Build history of the part. All positions in model axes, mm. Give positions to 0.01 mm unless a question says otherwise; leave off trailing zeros. Order: outer loops, then holes, each group sorted by start corner. A loop starts at its lowest first (then second) coordinate and runs counter-clockwise, first axis right, second up. Notation, with made-up numbers: (48, 31.25) - (91, 31.25) arc R5 cw to (91, 40.25) - close; hole circle Ø9 at (-36.75, 83.5). An arc over 180 degrees is marked (long way). Use a Markdown table: item, result. Add a question column.
(1) Slice it at D-D (x = 6). Write the cut outline in (y, z), then the cut area to 3 significant figures.
(2) Wall check: line 1 (Y direction, x = 0, z = -102.05); line 2 (X direction, y = 4.5, z = -101.05); line 3 (Y direction, x = -0.5, z = -100.25). Give the ranges that are in metal, low to high.
(3) Slice it at A-A (y = 0). Write the cut outline in (x, z), then the cut area to 3 significant figures.
(4) Mould opens along X. For faces 1 (the face through (11.444, -22.002, -102.028)), 2 (the face through (11, 6, -100)), 3 (the face through (14.5, 0, -102)) say: +X half, -X half, draft (parallel to the pull), parting line (faces both ways), or undercut.
(5) Slice it at C-C (y = -10). Write the cut outline in (x, z).
(6) Flat gauge pins, fed straight in: pin 1 (4 mm diameter, centred on x = 0, y = -16, fed in from +Z); pin 2 (2.5 mm diameter, centred on x = -16, y = 0, fed in from -Z); pin 3 (1.5 mm diameter, centred on x = -8, z = -102, fed in from -Y); pin 4 (2 mm diameter, centred on x = 10, z = -100.5, fed in from +Y). Where does each tip first touch, or does it go through?
from build123d import *

# Parameters (mm, degrees)
CYLINDER275_R               = 1.5
CYLINDER275_DEPTH           = 16
CYLINDER275_PLACEMENT_ANGLE = 67.5
CYLINDER273_R               = 1.5
CYLINDER273_DEPTH           = 16
CYLINDER273_PLACEMENT_ANGLE = 22.5
CYLINDER274_R               = 1.5
CYLINDER274_DEPTH           = 16
CYLINDER274_PLACEMENT_ANGLE = 112.5
CYLINDER272_R               = 1.5
CYLINDER272_DEPTH           = 16
CYLINDER272_PLACEMENT_ANGLE = 202.5
TUBE030_R                   = 24.8
TUBE030_R_2                 = 12
TUBE030_DEPTH               = 4


with BuildPart() as obj1:
    # Cylinder275 → Cylinder275 (new body)
    with BuildSketch(Plane.XY):
        Circle(CYLINDER275_R)
    extrude(amount=CYLINDER275_DEPTH)


with BuildPart() as obj1_1:
    # Cylinder275 placement: moved
    add(obj1.part.moved(Location((0, 16, 2))).rotate(Axis((0, 16, 2), (0, 0, -1)), CYLINDER275_PLACEMENT_ANGLE))


with BuildPart() as obj2:
    # Cylinder273 → Cylinder273 (new body)
    with BuildSketch(Plane.XY):
        Circle(CYLINDER273_R)
    extrude(amount=CYLINDER273_DEPTH)


with BuildPart() as obj2_1:
    # Cylinder273 placement: moved
    add(obj2.part.moved(Location((-16, 0, 2))).rotate(Axis((-16, 0, 2), (0, 0, 1)), CYLINDER273_PLACEMENT_ANGLE))


with BuildPart() as obj3:
    # Cylinder274 → Cylinder274 (new body)
    with BuildSketch(Plane.XY):
        Circle(CYLINDER274_R)
    extrude(amount=CYLINDER274_DEPTH)


with BuildPart() as obj3_1:
    # Cylinder274 placement: moved
    add(obj3.part.moved(Location((0, -16, 2))).rotate(Axis((0, -16, 2), (0, 0, 1)), CYLINDER274_PLACEMENT_ANGLE))


with BuildPart() as compound233:
    # Cylinder272 → Cylinder272 (new body)
    with BuildSketch(Plane.XY):
        Circle(CYLINDER272_R)
    extrude(amount=CYLINDER272_DEPTH)


with BuildPart() as compound233_1:
    # Cylinder272 placement: moved
    add(compound233.part.moved(Location((16, 0, 2))).rotate(Axis((16, 0, 2), (0, 0, 1)), CYLINDER272_PLACEMENT_ANGLE))

    # Compound233: union obj1, obj2, obj3
    add(obj1_1.part)
    add(obj2_1.part)
    add(obj3_1.part)


with BuildPart() as compound233_2:
    # Compound233 placement: moved
    add(compound233_1.part.moved(Location((0, 0, -117))))


with BuildPart() as cut124:
    # Tube030 → Tube030 (new body)
    with BuildSketch(Plane.XY.offset(-103)):
        Circle(TUBE030_R)
        Circle(TUBE030_R_2, mode=Mode.SUBTRACT)
    extrude(amount=TUBE030_DEPTH)

    # Cut124: cut Compound233
    add(compound233_2.part, mode=Mode.SUBTRACT)


with BuildPart() as cut124_1:
    # Cut124 placement: moved
    add(cut124.part.moved(Location((0, 0, -1))))


solid = cut124_1.part
Solution:
| question | item | result |
|---|---|---|
| 1 | outline | (-24.06, -104) - (-10.39, -104) - (-10.39, -100) - (-24.06, -100) - close; (10.39, -104) - (24.06, -104) - (24.06, -100) - (10.39, -100) - close |
| 1 | area | 109 mm2 |
| 2 | line 1 | -24.8 to -17.5, -14.5 to -12, 12 to 14.5, 17.5 to 24.8 |
| 2 | line 2 | -24.39 to -11.12, 11.12 to 24.39 |
| 2 | line 3 | -24.79 to -17.41, -14.59 to -11.99, 11.99 to 14.59, 17.41 to 24.79 |
| 3 | outline | (-24.8, -104) - (-17.5, -104) - (-17.5, -100) - (-24.8, -100) - close; (-14.5, -104) - (-12, -104) - (-12, -100) - (-14.5, -100) - close; (12, -104) - (14.5, -104) - (14.5, -100) - (12, -100) - close; (17.5, -104) - (24.8, -104) - (24.8, -100) - (17.5, -100) - close |
| 3 | area | 78.4 mm2 |
| 4 | face 1 | parting line |
| 4 | face 2 | draft |
| 4 | face 3 | undercut |
| 5 | outline | (-22.69, -104) - (-6.63, -104) - (-6.63, -100) - (-22.69, -100) - close; (6.63, -104) - (22.69, -104) - (22.69, -100) - (6.63, -100) - close |
| 6 | pin 1 | z = -100 |
| 6 | pin 2 | through |
| 6 | pin 3 | y = -23.72 |
| 6 | pin 4 | y = 23.11 |
